Design review of the part built by this model. Coordinates are the model's own, in mm. A direction names the side the tool comes from. Coordinates: 2 decimals unless noted, no trailing zeros. Write each loop counter-clockwise with the first axis right and the second up, starting at its lowest first coordinate (ties: lowest second). Pieces come first, ordered by that corner, then holes. Notation, with made-up numbers: (75, 26) -> (99, 26) arc R22 cw to (99, 48) -> close; hole circle Ø8 at (32.25, 31). An arc over 180 degrees is marked (long way). One line per question, with ' | ' between items. Start each with the question number.
Q1. Wall thickness on probe 1 along Z at (x, y) = (-342.5, 793.5); probe 2 along Y at (x, z) = (34, -331.5): over which ranges is each line inside the solid? List them lowest first.
Q2. Add section B-B on x = -17. State the section outline as (y, z) points, and give its area (3 significant figures).
Q3. Add section C-C on z = 101. State the section outline as (x, y) points.
Q4. For faces 5 (the flat face through (-352.15, 740, -433)), 6 (the flat face through (386.284, 740, -433)), 7 (the flat face through (-312.933, 740, -433)), 8 (the flat face through (-333, 740, -416.631)), 9 (the flat face through (-7, -5, -6)), list the 3-axis set-ups (+Z, -Z, +X, -X, +Y, -Y) from which the entire face can be reached by the end or side of a thin tool; tool diameter is ignored.
Q5. Add section A-A on y = 1188. State the section outline as (x, z) points, and give its area (3 significant figures).
Q6. For P1, Ø10, axis at y = 584.5, z = 440, coming from the +X side; P2, Ø10, axis at y = 971.5, z = 433.5, coming from the -X side; P3, Ø4, axis at x = -189, z = 195.5, coming from the +Y side, all flat-tipped, find the tip position at first contact; note any pin that passes through.
Q7. Draft analysis for pull direction Z (two halves, no side actions). For faces 1 (the flat face through (366, 740, -416.631)), 2 (the flat face through (-336, 749, -450)), 3 (the flat face through (-336, 749, 450)), 4 (the flat face through (386.284, 740, 434)), state which applies: pulls with the +Z half, pulls with the -Z half, needs draft (parallel to the pull), parting line crosses it, or undercut.
from build123d import *

# Parameters (mm, degrees)
SKETCH1_W           = 1000
SKETCH1_H           = 900
BOSS_EXTRUDE1_DEPTH = 5
SKETCH2_W           = 39.21699111
SKETCH2_H           = 33.368988095
BOSS_EXTRUDE2_DEPTH = 1500
FILLET1_R           = 10


with BuildPart() as part:
    # Sketch1 → Boss-Extrude1 (new, symmetric)
    with BuildSketch(Plane(origin=(0, 0, 0), x_dir=(1, 0, 0), z_dir=(0, 1, 0))):
        Rectangle(SKETCH1_W, SKETCH1_H)
    extrude(amount=BOSS_EXTRUDE1_DEPTH, both=True)

    # Sketch2 → Boss-Extrude2 (add)
    with BuildSketch(Plane(origin=(0, 5, 0), x_dir=(1, 0, 0), z_dir=(0, 1, 0))):
        with Locations((-332.541820244, -433.315505953)):
            Rectangle(SKETCH2_W, SKETCH2_H)
        with Locations((366.675170866, -433.315505953)):
            Rectangle(SKETCH2_W, SKETCH2_H)
        with Locations((366.675170866, 433.315505953)):
            Rectangle(SKETCH2_W, SKETCH2_H)
        with Locations((-332.541820244, 433.315505953)):
            Rectangle(SKETCH2_W, SKETCH2_H)
    extrude(amount=BOSS_EXTRUDE2_DEPTH)

    # Fillet1
    fillet1_edges = [part.edges().sort_by_distance(p)[0] for p in [
        (-352.150315799, 1505, 433.315505952),
        (-332.541820244, 1505, 450),
        (-312.933324689, 1505, 433.315505952),
        (-332.541820244, 1505, 416.631011905),
        (347.066675311, 1505, 433.315505952),
        (366.675170866, 1505, 450),
        (386.283666421, 1505, 433.315505952),
        (366.675170866, 1505, 416.631011905),
        (366.675170866, 1505, -450),
        (347.066675311, 1505, -433.315505952),
        (366.675170866, 1505, -416.631011905),
        (386.283666421, 1505, -433.315505952),
        (-332.541820244, 1505, -450),
        (-352.150315799, 1505, -433.315505952),
        (-332.541820244, 1505, -416.631011905),
        (-312.933324689, 1505, -433.315505952),
    ]]
    fillet(fillet1_edges, radius=FILLET1_R)


solid = part.part
Output values:
1) probe 1: z = -450 to -416.63, 416.63 to 450 | probe 2: y = -5 to 5
2) outline: (-5, -450) -> (5, -450) -> (5, 450) -> (-5, 450) -> close | area: 9,000 mm2
3) outline: (-500, -5) -> (500, -5) -> (500, 5) -> (-500, 5) -> close
4) face 5: +Z, -Z, -X, +Y | face 6: +Z, -Z, +X, +Y | face 7: +Z, -Z, +Y | face 8: +X, -X, +Y | face 9: +Z, -Z, +X, -X, -Y
5) outline: (-352.15, -450) -> (-312.93, -450) -> (-312.93, -416.63) -> (-352.15, -416.63) -> close; (-352.15, 416.63) -> (-312.93, 416.63) -> (-312.93, 450) -> (-352.15, 450) -> close; (347.07, -450) -> (386.28, -450) -> (386.28, -416.63) -> (347.07, -416.63) -> close; (347.07, 416.63) -> (386.28, 416.63) -> (386.28, 450) -> (347.07, 450) -> close | area: 5,230 mm2
6) P1: stops at x = 386.28 | P2: stops at x = -352.15 | P3: stops at y = 5
7) face 1: undercut | face 2: pulls with the -Z half | face 3: pulls with the +Z half | face 4: needs draft
